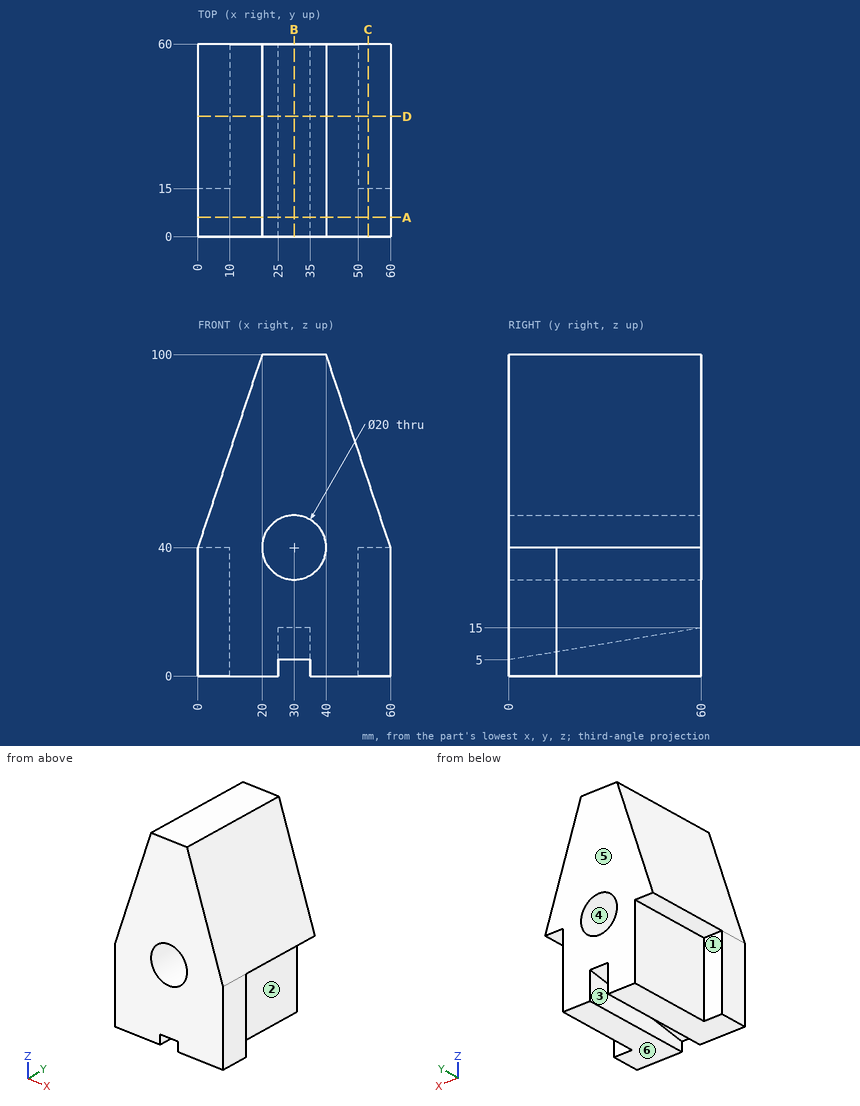
Could you check a few things on this drawing? It's one solid part, dimensions in mm from its lowest x, y, z. A direction names the side the tool comes from. Round coordinates to 2 decimals unless told otherwise and drop trailing zeros. Order: outer loops, then holes, each group sorted by start corner. A loop starts at its lowest first (then second) coordinate and runs counter-clockwise, first axis right, second up. Notation, with made-up numbers: M -9,56.5 L 25,56.5 A32 ccw 25,87.5 Z; hole C 35,-34.75 d7. An arc over 180 degrees is marked long. Return JSON: item names as keys, results as strings. Group by question number.
1. On a 3-axis mill with a long thin cutter (end or side, diameter ignored), from which of +Z, -Z, +X, -X, +Y, -Y can I reach the whole of each face in a straight line? I mean the marked faces 1, 2 and 3. Say none if no direction works.
2. If we section it at B-B on x = 30: List the corners of the cut face in (y, z) for me.
3. If we section it at A-A on y = 6: List the corners of the cut face in (x, z) for me.
4. Please list where these lines run through material, in increasing order: probe 1 along Z at (x, y) = (37, 14); probe 2 along Z at (x, y) = (30, 28.5); probe 3 along Y at (x, z) = (56, 29.5).
5. I'm going to push flat-ended pins straight in: pin 1 Ø4.5 at (y, z) = (17.5, 4) entering from -X; pin 2 Ø3 at (x, z) = (6.5, 18.5) entering from +Y; pin 3 Ø4.5 at (y, z) = (41, 8) entering from +X. Where does each tip first touch, or does it pass through?
6. If we mould it in two halves opening along Z, with no side actions, what happens to the marked faces 4, 5 and 6? For each: pulls with the +Z half, pulls with the -Z half, needs draft (parallel to the pull), parting line crosses it, or undercut.
7. If we section it at D-D on y = 37.5: List the corners of the cut face in (x, z) for me, then the cut area to 3 significant figures.
8. If we section it at C-C on x = 53: List the corners of the cut face in (y, z) for me.
Reply:
{
 "1": {"face 1": "-Z, -X, +Y", "face 2": "-Z, +X, +Y", "face 3": "-Z, +Y"},
 "2": {"outline": "M 0,5 L 60,15 L 60,30 L 0,30 Z; M 0,50 L 60,50 L 60,100 L 0,100 Z"},
 "3": {"outline": "M 0,0 L 25,0 L 25,6 L 35,6 L 35,0 L 60,0 L 60,40 L 40,100 L 20,100 L 0,40 Z; hole C 30,40 d20"},
 "4": {"probe 1": "0 to 32.86, 47.14 to 100", "probe 2": "9.75 to 30, 50 to 100", "probe 3": "0 to 15"},
 "5": {"pin 1": "x = 10", "pin 2": "y = 15", "pin 3": "x = 50"},
 "6": {"face 4": "undercut", "face 5": "needs draft", "face 6": "pulls with the -Z half"},
 "7": {"outline": "M 0,40 L 10,40 L 10,0 L 25,0 L 25,11.25 L 35,11.25 L 35,0 L 50,0 L 50,40 L 60,40 L 40,100 L 20,100 Z; hole C 30,40 d20", "area": "3,570 mm^2"},
 "8": {"outline": "M 0,0 L 15,0 L 15,40 L 60,40 L 60,61 L 0,61 Z"}
}
